Source: CAD feature listing. Evaluate the final solid. Frame: model axes, mm. A direction names the side the tool comes from. Coordinates: 2 decimals unless noted, no trailing zeros. Loops run counter-clockwise (first coordinate to the right, second up) from the corner with the lowest first, then second, coordinate; pieces in that order, holes last.
Item 1: Reachability of faces 1 (the cylindrical face through (-5.4, -24.4, 3.5)), 2 (the cylindrical face through (-6.4, 10.933, 0.281)), 3 (the flat face through (12, -65.694, 2)), 4 (the cylindrical face through (-2.21, -24.2, 3.55)), 5 (the cylindrical face through (6.33, -63.266, 0.451)) from +Z, -Z, +X, -X, +Y, -Y: full face, straight path, thin tool, end or side. Return the list, or none.
Item 2: Line query: probe 1 along X at (y, z) = (-58.5, 2.5); probe 2 along Y at (x, z) = (10.5, 3.35); probe 3 along Y at (x, z) = (15, 3.55). Output: solid intervals per line, ascending.
Item 3: Section query B-B, the plane x = 6. Return the cut outline in (y, z).
Item 4: Section query A-A, the plane y = -54. Return the cut outline in (x, z).
Item 5: Pin query (flat end, axial travel): pin 1 Ø1 at (y, z) = (-4.5, 2.5) entering from -X; pin 2 Ø0.8 at (x, z) = (-6.5, 2) entering from -Y; pin 3 Ø0.8 at (x, z) = (8, 2) entering from -Y. Return the tip coordinate at first contact, or that it passes through.
Item 6: Pull-direction query (Y, two-part tool) for faces 6 (the flat face through (10.218, -67, 2)), 7 (the cylindrical face through (-6.8, 13.88, 0.45)), 8 (the cylindrical face through (6.33, -63.266, 3.549)), 9 (the cylindrical face through (-6.4, 10.933, 3.719)); classes: +Y half, -Y half, draft (parallel to the pull), parting line (faces both ways), or undercut.
```python
from build123d import *

# Parameters (mm, degrees)
F1_DEPTH = 4
F2_R     = 1.5


# Not quite as in the source:
# - ends of sketch curves that miss each other by under 0.0002 mm in the source are joined


with BuildPart() as f1:
    # F0 (on Top) → F1 (new body)
    with BuildSketch(Plane.XY):
        with BuildLine():
            Line((-5.7822973108, 10.3064593036), (-5.7822973108, 0))
            Line((-5.7822973108, 0), (-5.7822973108, -59.6935572128))
            ThreePointArc((-5.7822973108, -59.6935572128), (-4.6107244356, -62.5219843376), (-1.7822973108, -63.6935572128))
            Line((-1.7822973108, -63.6935572128), (14.2177026892, -63.6935572128))
            Line((14.2177026892, -63.6935572128), (14.2177026892, -65.6935572128))
            Line((14.2177026892, -65.6935572128), (10.2177026892, -65.6935572128))
            Line((10.2177026892, -65.6935572128), (10.2177026892, -67.6935572128))
            Line((10.2177026892, -67.6935572128), (18.2177026892, -67.6935572128))
            Line((18.2177026892, -67.6935572128), (18.2177026892, -59.6935572128))
            Line((18.2177026892, -59.6935572128), (-1.7822973108, -59.6935572128))
            Line((-1.7822973108, -59.6935572128), (-1.7822973108, 10.3064427872))
            ThreePointArc((-1.7822973108, 10.3064427872), (-2.9538701861, 13.1348699119), (-5.7822973108, 14.3064427872))
            Line((-5.7822973108, 14.3064427872), (-7.7880364463, 14.3064427872))
            ThreePointArc((-7.7880364463, 14.3064427872), (-9.2042805699, 13.7186228687), (-9.7880281881, 12.3006953697))
            ThreePointArc((-9.7880281881, 12.3006953697), (-9.2002165753, 10.8902151801), (-7.7880364938, 10.3064593036))
            Line((-7.7880364938, 10.3064593036), (-5.7822973108, 10.3064593036))
        make_face()
    extrude(amount=F1_DEPTH)

    # F2
    f2_edges = [f1.edges().sort_by_distance(p)[0] for p in [
        (-5.782297, -24.693549, 4),
        (-1.782297, -24.693557, 4),
        (-2.95387, 13.13487, 4),
        (-6.785167, 14.306443, 4),
        (-9.204281, 13.718623, 4),
        (-9.200211, 10.890209, 4),
        (-6.785167, 10.306459, 4),
        (-1.782297, -24.693557, 0),
        (-2.95387, 13.13487, 0),
        (-6.785167, 14.306443, 0),
        (-9.204281, 13.718623, 0),
        (-9.200211, 10.890209, 0),
        (-6.785167, 10.306459, 0),
        (-5.782297, -24.693549, 0),
    ]]
    fillet(f2_edges, radius=F2_R)


solid = f1.part
```
Verdict:
1. face 1: +Z, -X, -Y
1. face 2: -Z, -X, -Y
1. face 3: +Z, -Z, -X
1. face 4: +Z, +X, +Y
1. face 5: -Z, -X
2. probe 1: x = -5.78 to -1.78
2. probe 2: y = -67.69 to -65.69, -63.43 to -59.69
2. probe 3: y = -67.69 to -59.69
3. outline: (-63.69, 1.5) arc R1.5 ccw to (-62.19, 0) - (-59.69, 0) - (-59.69, 4) - (-62.19, 4) arc R1.5 ccw to (-63.69, 2.5) - close
4. outline: (-5.78, 1.5) arc R1.5 ccw to (-4.28, 0) - (-3.28, 0) arc R1.5 ccw to (-1.78, 1.5) - (-1.78, 2.5) arc R1.5 ccw to (-3.28, 4) - (-4.28, 4) arc R1.5 ccw to (-5.78, 2.5) - close
5. pin 1: stops at x = -5.78
5. pin 2: stops at y = 10.31
5. pin 3: stops at y = -63.69
6. face 6: draft
6. face 7: +Y half
6. face 8: undercut
6. face 9: -Y half
